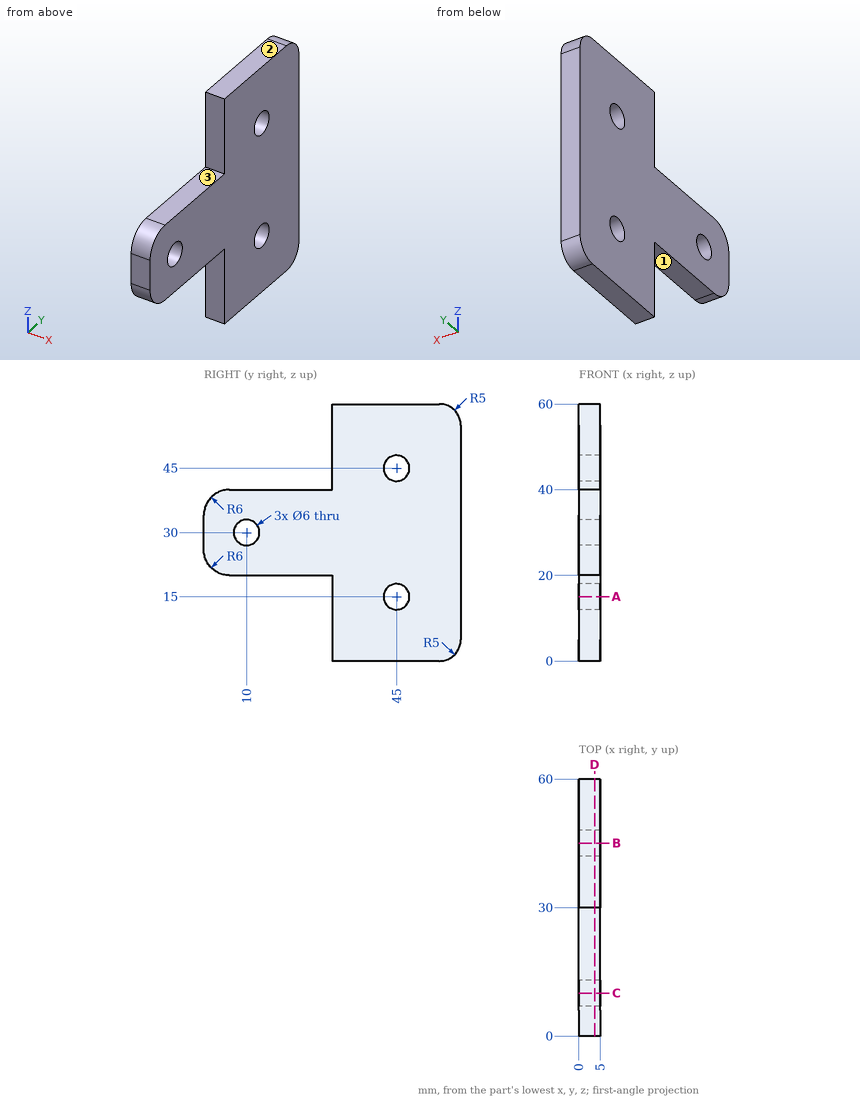
Verification items for this drawing (mm, ordinates from the low corner). A direction names the side the tool comes from. Coordinates: 2 decimals unless noted, no trailing zeros. Order: outer loops, then holes, each group sorted by start corner. A loop starts at its lowest first (then second) coordinate and runs counter-clockwise, first axis right, second up. Notation, with made-up numbers: M 53,-19.75 L 109,-19.75 A18 cw 109,-9.75 Z; hole C 56,-39.5 d2. An arc over 180 degrees is marked long. Answer as a JSON object with one key per item and string values.
Q1. Cross-section at C-C on y = 10. Record the cut outline in (x, z), and give its area (3 significant figures).
Results are:
{"outline": "M 0,20 L 5,20 L 5,27 L 0,27 Z; M 0,33 L 5,33 L 5,40 L 0,40 Z", "area": "70.0 mm²"}
Q2. Cross-section at A-A on z = 15. Record the cut outline in (x, y), and give its area (3 significant figures).
Results are:
{"outline": "M 0,30 L 5,30 L 5,42 L 0,42 Z; M 0,48 L 5,48 L 5,60 L 0,60 Z", "area": "120 mm²"}
Q3. Cross-section at B-B on y = 45. Record the cut outline in (x, z), and give its area (3 significant figures).
Results are:
{"outline": "M 0,0 L 5,0 L 5,12 L 0,12 Z; M 0,18 L 5,18 L 5,42 L 0,42 Z; M 0,48 L 5,48 L 5,60 L 0,60 Z", "area": "240 mm²"}
Q4. Scan lines: line 1 (Z direction, x = 2.85, y = 45); line 2 (Z direction, x = 2.95, y = 10); line 3 (Z direction, x = 3.8, y = 46). Record each from-to range of solid material in increasing order.
Results are:
{"line 1": "z = 0 to 12, 18 to 42, 48 to 60", "line 2": "z = 20 to 27, 33 to 40", "line 3": "z = 0 to 12.17, 17.83 to 42.17, 47.83 to 60"}
Q5. Cross-section at D-D on x = 3.7. Record the cut outline in (y, z).
Results are:
{"outline": "M 0,26 A6 ccw 6,20 L 30,20 L 30,0 L 55,0 A5 ccw 60,5 L 60,55 A5 ccw 55,60 L 30,60 L 30,40 L 6,40 A6 ccw 0,34 Z; hole C 10,30 d6; hole C 45,15 d6; hole C 45,45 d6"}
Q6. Depth check by flat-ended pin: pin 1 Ø2.5 at (x, y) = (3.5, 22) entering from -Z; pin 2 Ø1.5 at (x, z) = (2, 9) entering from -Y. Enter the tip coordinate at first touch or a pass-through.
Results are:
{"pin 1": "stops at z = 20", "pin 2": "stops at y = 30"}
Q7. Tool access check on the marked faces 1, 2 and 3. Record the directions out of +Z, -Z, +X, -X, +Y, -Y that give a thin tool (end or side, any length) a straight path to the whole face; none if there is none.
Results are:
{"face 1": "-Z, +X, -X, -Y", "face 2": "+Z, +X, -X, +Y, -Y", "face 3": "+Z, +X, -X, -Y"}
